Verification items for the finished model (mm, model axes). Face numbers are marked on the shaded views. A direction names the side the tool comes from. Round coordinates to 2 decimals unless told otherwise and drop trailing zeros. Write each loop counter-clockwise with the first axis right and the second up, starting at its lowest first coordinate (ties: lowest second). Pieces come first, ordered by that corner, then holes. Notation, with made-up numbers: (36, -28) -> (64, -28) arc R9 cw to (64, -13) -> close; hole circle Ø2 at (-36, 15.25). An arc over 180 degrees is marked (long way). Answer as a JSON object with one key per item and string values. Group by question number.
(1) Gauge pin test, flat ends, axial feed: pin 1 Ø5 at (x, y) = (126.5, 68.5) entering from +Z; pin 2 Ø1.5 at (y, z) = (96.5, 13.5) entering from -X; pin 3 Ø12 at (x, y) = (81, 78.5) entering from -Z. Record the tip position at first contact, or that the pin passes through.
(2) Sectioned sample at C-C on y = 60. Record the cut outline in (x, z), and give its area (3 significant figures).
(3) Sectioned sample at D-D on x = 111.5. Record the cut outline in (y, z), and give its area (3 significant figures).
(4) Sectioned sample at A-A on x = 8. Record the cut outline in (y, z), and give its area (4 significant figures).
(5) Sectioned sample at B-B on y = 44. Record the cut outline in (x, z), and give its area (3 significant figures).
(6) Scan lines: L1, parallel to Y at x = 1.45, z = 8; L2, parallel to Y at x = 123.4, z = 10.75; L3, parallel to X at y = 81.5, z = 7. Record each from-to range of solid material in increasing order. Write a range as from..to.
(7) Set-up check for the marked faces 4, 5 and 6: record each of +Z, -Z, +X, -X, +Y, -Y from which the full face is reachable in a straight line by a thin tool's end or side.
(8) Draft check along X on the marked faces 1, 2 and 3. Enter one of: released by +X, released by -X, zero draft, split by the parting line, or undercut.
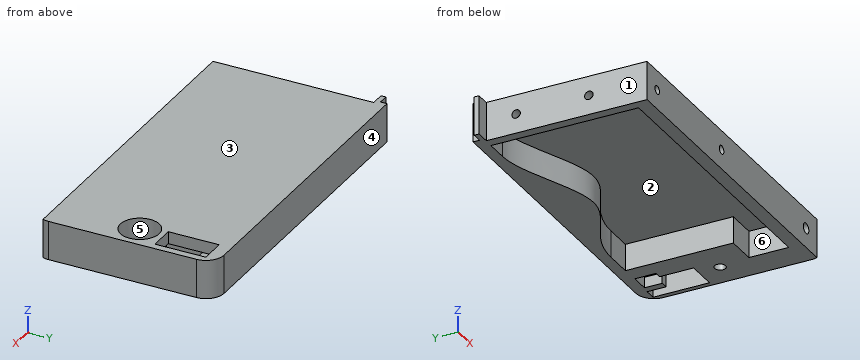
```python
from build123d import *

# Parameters (mm, degrees)
SKETCH_R        = 2.25
PAD_DEPTH       = 16
POCKET_DEPTH    = 21
SKETCH002_R     = 1.75
POCKET001_DEPTH = 23
SKETCH003_R     = 1.75
SKETCH003_R_2   = 2.15
POCKET002_DEPTH = 46
SKETCH005_R     = 8
POCKET004_DEPTH = 5
POCKET005_DEPTH = 4.4
SKETCH007_W     = 10.5
SKETCH007_H     = 21
POCKET006_DEPTH = 5
POCKET007_DEPTH = 18


with BuildPart() as part:
    # Sketch → Pad (new body)
    with BuildSketch(Plane.XY):
        with BuildLine():
            Line((0, 36), (75.6, 36))
            Line((75.6, 36), (133.571068, 36))
            ThreePointArc((133.571068, 36), (133.891989, 37.231735), (134, 38.5))
            Line((134, 38.5), (134, 99.5))
            ThreePointArc((134, 99.5), (131.803301, 104.803301), (126.5, 107))
            Line((126.5, 107), (-1.5, 107))
            Line((-1.5, 107), (-1.5, 104.3))
            Line((-1.5, 104.3), (-5.7, 104.3))
            Line((-5.7, 104.3), (-5.7, 102.3))
            Line((-5.7, 102.3), (0, 102.3))
            Line((0, 102.3), (0, 36))
        make_face()
        with Locations((123.4, 70.6)):
            Circle(SKETCH_R, mode=Mode.SUBTRACT)
    extrude(amount=PAD_DEPTH)

    # Sketch001 (on DatumPlane) → Pocket (cut)
    with BuildSketch(Plane.XY.offset(11)):
        with BuildLine():
            Line((13.289069, 102.5), (4, 102.5))
            Line((4, 102.5), (4, 41.6))
            Line((4, 41.6), (80, 41.6))
            Line((80, 41.6), (122, 41.6))
            Line((122, 41.6), (122, 58))
            Line((122, 58), (109.7, 58))
            Line((109.7, 58), (109.7, 102.5))
            Line((109.7, 102.5), (98.331885, 102.5))
            add(Edge.make_bspline(
                [(13.289069, 102.5), (27.487875, 102.5), (63.575842, 75.600151), (81.110251, 102.5), (98.331885, 102.5)],
                knots=[0, 0, 0, 0, 0.5, 1, 1, 1, 1], degree=3))
        make_face()
        Polygon((128.6, 101.8), (131, 101.8), (131, 79.9), (120.7, 79.9), (120.7, 93.6), (120.7, 93.9), (124.3, 93.9), (128.6, 93.9), align=None)
    extrude(amount=-POCKET_DEPTH, mode=Mode.SUBTRACT)

    # Sketch002 → Pocket001 (cut)
    with BuildSketch(Plane.YZ):
        with Locations((12, 8)):
            Circle(SKETCH002_R)
        with Locations((60, 8)):
            Circle(SKETCH002_R)
        with Locations((90, 8)):
            Circle(SKETCH002_R)
    extrude(amount=POCKET001_DEPTH, mode=Mode.SUBTRACT)

    # Sketch003 → Pocket002 (cut)
    with BuildSketch(Plane.XZ):
        with Locations((58.6, 8)):
            Circle(SKETCH003_R)
        with Locations((8, 8)):
            Circle(SKETCH003_R)
        with Locations((125, 8)):
            Circle(SKETCH003_R_2)
    extrude(amount=-POCKET002_DEPTH, mode=Mode.SUBTRACT)

    # Sketch005 (on DatumPlane) → Pocket004 (cut, symmetric)
    with BuildSketch(Plane.XY.offset(11)):
        with Locations((123.4, 70.6)):
            Circle(SKETCH005_R)
    extrude(amount=POCKET004_DEPTH, both=True, mode=Mode.SUBTRACT)

    # Sketch006 → Pocket005 (cut)
    with BuildSketch(Plane.XY):
        Polygon((116.7, 102.3), (124.3, 102.3), (124.3, 93.9), (124.3, 93.6), (120.7, 93.6), (116.7, 93.6), align=None)
    extrude(amount=POCKET005_DEPTH, mode=Mode.SUBTRACT)

    # Sketch007 (on DatumPlane) → Pocket006 (cut)
    with BuildSketch(Plane.XY.offset(11)):
        with Locations((125.75, 91.3)):
            Rectangle(SKETCH007_W, SKETCH007_H)
    extrude(amount=POCKET006_DEPTH, mode=Mode.SUBTRACT)

    # Sketch008 (on DatumPlane) → Pocket007 (cut)
    with BuildSketch(Plane.XY.offset(11)):
        Polygon((127.328613, 102.8), (132, 102.8), (132, 79.494476), (119.5, 79.494476), (119.5, 94.960373), (127.328613, 94.960373), align=None)
    extrude(amount=-POCKET007_DEPTH, mode=Mode.SUBTRACT)


solid = part.part
```
Computed values:
{
 "1": {"pin 1": "z = 6", "pin 2": "x = 0", "pin 3": "z = 11"},
 "2": {"outline": "(0, 0) -> (4, 0) -> (4, 6.25) -> (0, 6.25) -> close; (0, 9.75) -> (4, 9.75) -> (4, 11) -> (109.7, 11) -> (109.7, 0) -> (134, 0) -> (134, 16) -> (0, 16) -> close", "area": "967 mm2"},
 "3": {"outline": "(36, 0) -> (41.6, 0) -> (41.6, 11) -> (58, 11) -> (58, 0) -> (107, 0) -> (107, 16) -> (36, 16) -> close", "area": "956 mm2"},
 "4": {"outline": "(36, 0) -> (41.6, 0) -> (41.6, 6.25) -> (36, 6.25) -> close; (36, 9.75) -> (41.6, 9.75) -> (41.6, 11) -> (102.5, 11) -> (102.5, 0) -> (107, 0) -> (107, 16) -> (36, 16) -> close", "area": "446.5 mm2"},
 "5": {"outline": "(0, 0) -> (4, 0) -> (4, 11) -> (122, 11) -> (122, 0) -> (134, 0) -> (134, 16) -> (0, 16) -> close; hole circle Ø4.3 at (125, 8)", "area": "831 mm2"},
 "6": {"L1": "36..58.25, 61.75..88.25, 91.75..107", "L2": "36..62.6, 78.6..79.49, 94.96..107", "L3": "0..4, 109.7..119.5, 132..134"},
 "7": {"face 4": "+Z, -Z, +X, -X, +Y", "face 5": "+Z", "face 6": "-Z"},
 "8": {"face 1": "released by -X", "face 2": "undercut", "face 3": "zero draft"}
}
